```python
from build123d import *

# Parameters (mm, degrees)
F1_DEPTH = 9.525
F2_R     = 2.54
F3_R     = 5.08
F4_R     = 1.26999


# Not quite as in the source:
# - a fillet or chamfer is up to 0.001 mm smaller than in the source, because OpenCascade refuses the exact size


with BuildPart() as f1:
    # F0 (on Top) → F1 (new body)
    with BuildSketch(Plane.XY):
        Polygon((-28.575, 0), (0, 0), (0, -48.26), (17.78, -48.26), (17.78, -41.275), (15.24, -41.275), (15.24, -45.72), (2.54, -45.72), (2.54, 2.54), (-31.115, 2.54), (-31.115, -22.86), (-28.575, -22.86), align=None)
    extrude(amount=F1_DEPTH)

    # F2
    f2_edges = [f1.edges().sort_by_distance(p)[0] for p in [
        (15.24, -45.72, 4.7625),
        (2.54, -45.72, 4.7625),
        (-28.575, 0, 4.7625),
        (0, 0, 4.7625),
    ]]
    fillet(f2_edges, radius=F2_R)

    # F3
    f3_edges = [f1.edges().sort_by_distance(p)[0] for p in [
        (17.78, -48.26, 4.7625),
        (0, -48.26, 4.7625),
        (2.54, 2.54, 4.7625),
        (-31.115, 2.54, 4.7625),
    ]]
    fillet(f3_edges, radius=F3_R)

    # F4 (radius 1.27 in the source; OpenCascade refuses exactly that, so slightly less here)
    f4_edges = [f1.edges().sort_by_distance(p)[0] for p in [
        (-31.115, -22.86, 4.7625),
        (-28.575, -22.86, 4.7625),
        (15.24, -41.275, 4.7625),
        (17.78, -41.275, 4.7625),
    ]]
    fillet(f4_edges, radius=F4_R)


solid = f1.part
```
Part model, mm, in its own coordinate system. A direction names the side the tool comes from. Coordinates: 2 decimals unless noted, no trailing zeros. Order: outer loops, then holes, each group sorted by start corner. A loop starts at its lowest first (then second) coordinate and runs counter-clockwise, first axis right, second up. Notation, with made-up numbers: (76.5, 86) -> (95.5, 86) arc R20 ccw to (95.5, 93) -> close; hole circle Ø9 at (89, -6). An arc over 180 degrees is marked (long way). Put each result on its own line as item: value. Start each with the question number.
(1) Probe line 1 along X through (y, z) = (-12, 6.5) (3 decimals); line 2 along X through (y, z) = (-42.5, 7.5); line 3 along Y through (x, z) = (-11, 3.25). List the from-to ranges inside material, lowest first. Write a range as [from, to].
(2) Mould opens along X. For faces 4 (the face through (-30.73, -22.5, 4.83)), 5 (the face through (16.252, -46.811, 4.829)), 6 (the face through (-14, 0, 5)) say: pulls with the +X half, pulls with the -X half, needs draft (parallel to the pull), parting line crosses it, or undercut.
(3) Pin check, flat tips, straight feed: pin 1 Ø5 at (x, z) = (-19.5, 4.5) entering from -Y; pin 2 Ø4 at (y, z) = (-15, 3.5) entering from +X; pin 3 Ø4 at (x, z) = (10, 7) entering from +Y. Stop position of each tip, or through.
(4) Which spindle directions (+Z, -Z, +X, -X, +Y, -Y) get a long thin tool onto all of the face, cutting with end or side? Do faces 1 (the face through (0, -23, 5)), 2 (the face through (14.516, -44.956, 4.829)), 3 (the face through (0.5, -19, 0)). Say none if no direction does.
(5) Band-saw the part on C-C (y = -26.5). Give the cut face in (x, z) (3 decimals), then the cut area to 3 significant figures.
(6) Band-saw the part on A-A (y = -18). Give the cut face in (x, z) (3 decimals), then the cut area to 3 significant figures.
Determined:
1. line 1: x = [-31.115, -28.575], [0, 2.54]
1. line 2: x = [0, 2.54], [15.24, 17.78]
1. line 3: y = [0, 2.54]
2. face 4: pulls with the -X half
2. face 5: pulls with the +X half
2. face 6: undercut
3. pin 1: stops at y = 0
3. pin 2: stops at x = 2.54
3. pin 3: stops at y = -45.72
4. face 1: +Z, -Z, -Y
4. face 2: +Z, -Z, +Y
4. face 3: -Z, +X, -X, +Y, -Y
5. outline: (0, 0) -> (2.54, 0) -> (2.54, 9.525) -> (0, 9.525) -> close
5. area: 24.2 mm²
6. outline: (-31.115, 0) -> (-28.575, 0) -> (-28.575, 9.525) -> (-31.115, 9.525) -> close; (0, 0) -> (2.54, 0) -> (2.54, 9.525) -> (0, 9.525) -> close
6. area: 48.4 mm²
